Autodesk Inventor part; units mm, degrees
ref_plane "YZ Plane" through (0, 0, 0) normal (1, 0, 0) x (0, 1, 0)
ref_plane "XZ Plane" through (0, 0, 0) normal (0, 1, 0) x (-1, 0, 0)
ref_plane "XY Plane" through (0, 0, 0) normal (0, 0, 1) x (1, 0, 0)
sketch "Sketch2" plane through (0, 0, 0) normal (0, 0, 1) x (1, 0, 0)
  line L0 (30, -30) -> (-30, -30)
  line L1 (-30, -30) -> (-30, 30)
  line L2 (-30, 30) -> (30, 30)
  line L3 (30, 30) -> (30, -30)
  line L4 (30, -30) -> (-30, 30) construction
  line L5 (-30, -30) -> (30, 30) construction
  circle A0 centre (-20, 20) radius 3.25
  circle A1 centre (20, 20) radius 3.25
  circle A2 centre (-20, -20) radius 3.25
  circle A3 centre (20, -20) radius 3.25
  point P0 (0, 0)
  dimension "d0" = 60
  dimension "d1" = 60
  dimension "d13" = 6.5
  dimension "d14" = 6.5
  dimension "d15" = 6.5
  dimension "d16" = 6.5
  dimension "d17" = 10
  dimension "d19" = 10
  dimension "d20" = 10
  dimension "d21" = 10
extrude "Extrusion1" add sketch "Sketch2" along normal blind 4
sketch "Sketch5" plane through (0, 0, 0) normal (0, 1, 0) x (-1, 0, 0)
  line L0 (-30, 0) -> (30, 0) construction
  line L1 (30, 0) -> (30, 4) construction
  line L2 (-30, 4) -> (30, 4) construction
  line L3 (-30, 0) -> (-30, 4) construction
  line L4 (88.4744, 0) -> (-49.7457, 0) construction
  line L5 (-30, 0) -> (64.1719, -26.056)
  line L6 (66.687, -24.3976) -> (68.3165, -12.3976)
  line L7 (66.868, -10.2009) -> (30, 0)
  line L8 (30, 0) -> (-30, 0)
  arc A0 (68.3165, -12.3976) -> (66.868, -10.2009) centre (66.3347, -12.1284) ccw
  arc A1 (64.1719, -26.056) -> (66.687, -24.3976) centre (64.7052, -24.1284) ccw
  point P0 (66.3789, -26.6667)
  point P1 (68.5516, -10.6667)
  dimension "d26" = 100
  dimension "d31" = 40
  dimension "d32" = 2
  dimension "d37" = 16
extrude "Extrusion3" add sketch "Sketch5" along normal mid plane 4
fillet "Fillet1" radius 1 2 edges at (0, 2, 0) (0, -2, 0)
sketch "Sketch6" plane through (0, -2, 0) normal (0, -1, 0) x (1, 0, 0)
  line L0 (-33.6142, -1) -> (26.3858, -1) construction
  line L1 (-33.6142, -1) -> (-66.868, -10.2009) construction
  arc A0 (-66.868, -10.2009) -> (-68.3165, -12.3976) centre (-66.3347, -12.1284) ccw construction
  line L2 (-68.3165, -12.3976) -> (-66.687, -24.3976) construction
  arc A1 (-66.687, -24.3976) -> (-64.1719, -26.056) centre (-64.7052, -24.1284) ccw construction
  line L3 (-64.1719, -26.056) -> (26.3858, -1) construction
  point P0 (0, 0)
  point P1 (-57.7389, -15.9755)
  dimension "d34" = 16
  dimension "d35" = 8
  dimension "d36" = 10
hole "Hole1" at (-57.7389, -2, -15.9755) direction (0, 1, 0) diameter 8.5 depth 10
properties part number "P044_SupportCaméra"
Design review of the part built by this model. Coordinates are the model's own, in mm. A direction names the side the tool comes from. Coordinates: 2 decimals unless noted, no trailing zeros. Order: outer loops, then holes, each group sorted by start corner. A loop starts at its lowest first (then second) coordinate and runs counter-clockwise, first axis right, second up. Notation, with made-up numbers: M 22,88.5 L 73,88.5 A18 cw 73,96.5 Z; hole C 9,83.5 d5. An arc over 180 degrees is marked long. Answer as a JSON object with one key per item and string values. Group by question number.
1) Add section B-B, the plane y = -20. Write out the cut boundary in (x, z).
2) Wall thickness on L1, parallel to Y at x = -20, z = 1.7; L2, parallel to Y at x = -8, z = -1; L3, parallel to Z at x = -9, y = -23: over which ranges is each line inside the solid? List them lowest first.
3) Tool access review of faces 5 (the flat face through (0, 30, 2)), 6 (the flat face through (-31, -2, -11)), 7 (the flat face through (-31, 2, -11)): name each direction out of +Z, -Z, +X, -X, +Y, -Y from which nothing blocks a thin tool from reaching the whole face with its end or side.
4) Add section A-A, the plane z = 2.5. Write out the cut boundary in (x, y), then the cut area to 3 significant figures.
5) For pin 1 (13.5 mm diameter, centred on x = -57.74, z = -15.98, fed in from -Y); pin 2 (10.5 mm diameter, centred on x = 20, y = 20, fed in from -Z); pin 3 (10 mm diameter, centred on x = 8, y = 1.5, fed in from -Z); pin 4 (5 mm diameter, centred on x = 20, y = -20, fed in from -Z), all flat-tipped, find the tip position at first contact; note any pin that passes through.
6) Mouldability with a two-part tool opening along X and no side actions: class faces 1 (the cylindrical face through (-23.247, -20.143, 1.972)), 2 (the flat face through (-67.49, -0.03, -18.48)), 3 (the flat face through (0, -16, 0)), 4 (the cylindrical face through (-23.247, 19.857, 1.972)) as pulls with the +X half, pulls with the -X half, needs draft (parallel to the pull), parting line crosses it, or undercut.
7) Add section D-D, the plane x = 1. Write out the cut boundary in (y, z), then the cut area to 3 significant figures.
8) Add section C-C, the plane x = 20. Write out the cut boundary in (y, z), then the cut area to 3 significant figures.
Computed values:
{
 "1": {"outline": "M -30,0 L -23.25,0 L -23.25,4 L -30,4 Z; M -16.75,0 L 16.75,0 L 16.75,4 L -16.75,4 Z; M 23.25,0 L 30,0 L 30,4 L 23.25,4 Z"},
 "2": {"L1": "y = -30 to -23.25, -16.75 to 16.75, 23.25 to 30", "L2": "y = -2 to 2", "L3": "z = 0 to 4"},
 "3": {"face 5": "+Z, -Z, +X, -X, +Y", "face 6": "-Z, +X, -X, -Y", "face 7": "-Z, +X, -X, +Y"},
 "4": {"outline": "M -30,-30 L 30,-30 L 30,30 L -30,30 Z; hole C -20,-20 d6.5; hole C -20,20 d6.5; hole C 20,-20 d6.5; hole C 20,20 d6.5", "area": "3,470 mm^2"},
 "5": {"pin 1": "stops at y = -2", "pin 2": "stops at z = 0", "pin 3": "stops at z = -7.47", "pin 4": "passes through"},
 "6": {"face 1": "undercut", "face 2": "pulls with the -X half", "face 3": "needs draft", "face 4": "undercut"},
 "7": {"outline": "M -30,0 L -3,0 A1 cw -2,-1 L -2,-8.02 L 2,-8.02 L 2,-1 A1 cw 3,0 L 30,0 L 30,4 L -30,4 Z", "area": "273 mm^2"},
 "8": {"outline": "M -30,0 L -23.25,0 L -23.25,4 L -30,4 Z; M -16.75,0 L -3,0 A1 cw -2,-1 L -2,-2.77 L 2,-2.77 L 2,-1 A1 cw 3,0 L 16.75,0 L 16.75,4 L -16.75,4 Z; M 23.25,0 L 30,0 L 30,4 L 23.25,4 Z", "area": "199 mm^2"}
}
